Input: part model. Units: mm. Frame: model coordinates. Face numbers are marked on the shaded views. Round coordinates to 2 decimals unless told otherwise and drop trailing zeros. Write each loop counter-clockwise with the first axis right and the second up, starting at its lowest first coordinate (ties: lowest second). Pieces come first, ordered by that corner, then holes. Notation, with made-up numbers: (-30, 82) -> (9, 82) arc R17 ccw to (9, 101) -> close; hole circle Ø2 at (17, -16). An arc over 180 degrees is marked (long way). Write item = value, one per line. Start each with the question number.
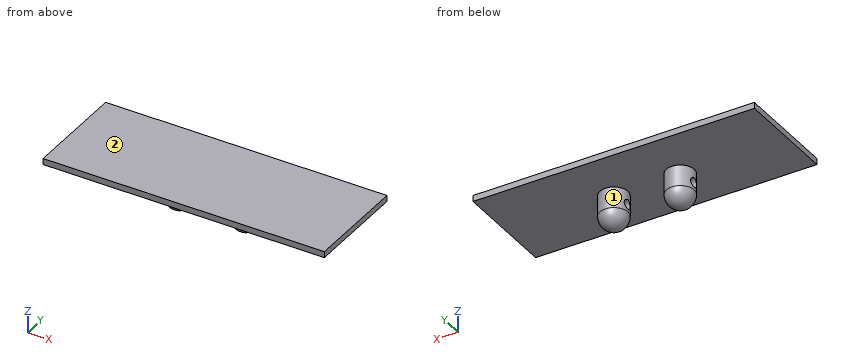
```python
from build123d import *

# Parameters (mm, degrees)
F0_W      = 88
F0_H      = 37
F1_DEPTH  = 1.75
F2_W      = 80.5
F2_H      = 29.5
F3_DEPTH  = 1.5
F4_R      = 4
F5_DEPTH  = 10
F6_R      = 4
F7_R      = 1.35
F8_DEPTH  = 88.001
F9_R      = 3
F10_DEPTH = 25


with BuildPart() as f1:
    # F0 (on Top) → F1 (new body)
    with BuildSketch(Plane.XY):
        with Locations((-44, 18.5)):
            Rectangle(F0_W, F0_H)
    extrude(amount=F1_DEPTH)

    # F2 (on face) → F3 (join)
    with BuildSketch(Plane.XY.offset(1.75)):
        with Locations((-44, 18.5)):
            Rectangle(F2_W, F2_H)
    extrude(amount=F3_DEPTH)

    # F4 (on face) → F5 (join)
    with BuildSketch(Plane(origin=(0, 0, 0), x_dir=(1, 0, 0), z_dir=(0, 0, -1))):
        with Locations((-53.5, -17.5)):
            Circle(F4_R)
        with Locations((-34.5, -17.5)):
            Circle(F4_R)
    extrude(amount=F5_DEPTH)

    # F6
    f6_edges = [f1.edges().sort_by_distance(p)[0] for p in [
        (-57.5, 17.5, -10),
        (-38.5, 17.5, -10),
    ]]
    fillet(f6_edges, radius=F6_R)

    # F7 (on face) → F8 (cut, through all)
    with BuildSketch(Plane.YZ):
        with Locations((17.5, -3.85)):
            Circle(F7_R)
    extrude(amount=-F8_DEPTH, mode=Mode.SUBTRACT)

    # F9
    f9_edges = [f1.edges().sort_by_distance(p)[0] for p in [
        (-88, 0, 0.875),
        (-88, 37, 0.875),
        (0, 37, 0.875),
        (0, 0, 0.875),
    ]]
    fillet(f9_edges, radius=F9_R)

    # F2 (on face) → F10 (intersect)
    with BuildSketch(Plane.XY.offset(1.75)):
        with Locations((-44, 18.5)):
            Rectangle(F2_W, F2_H)
    extrude(amount=-F10_DEPTH, mode=Mode.INTERSECT)


solid = f1.part
```
1. Section D-D (y = 8.5). Output: boundary loops of the cut face in (x, z).
2. Pin query (flat end, axial travel): P1, Ø5, axis at y = 27, z = -1, coming from the -X side; P2, Ø4, axis at x = -63.5, y = 11, coming from the -Z side; P3, Ø4.5, axis at y = 17.5, z = -3.85, coming from the -X side. Return the tip coordinate at first contact, or that it passes through.
3. Line query: line 1 along X through (y, z) = (19.75, -5); line 2 along X through (y, z) = (14.25, -5.75); line 3 along Y through (x, z) = (-54, -3.85). Output: solid intervals per line, ascending.
4. Section C-C (z = -3.85). Output: boundary loops of the cut face in (x, y).
5. Section B-B (z = -0.75). Output: boundary loops of the cut face in (x, y).
6. Mould query, pull axis X, two halves, no side actions, for the marked faces 1 and 2. Classes: pulls with the +X half, pulls with the -X half, needs draft (parallel to the pull), parting line crosses it, or undercut.
7. Section A-A (x = -34.5). Output: boundary loops of the cut face in (y, z), then the cut area to 3 significant figures.
Check sheet entries:
q1.outline = (-84.25, 0) -> (-3.75, 0) -> (-3.75, 1.75) -> (-84.25, 1.75) -> close
q2.P1 = -84.25
q2.P2 = 0
q2.P3 = -57.5
q3.line_1 = -56.81 to -50.19, -37.81 to -31.19
q3.line_2 = -55.83 to -51.17, -36.83 to -32.17
q3.line_3 = 13.53 to 16.15, 18.85 to 21.47
q4.outline = (-57.27, 16.15) arc R4 ccw to (-49.73, 16.15) -> close; (-57.27, 18.85) -> (-49.73, 18.85) arc R4 ccw to start; (-38.27, 16.15) arc R4 ccw to (-30.73, 16.15) -> close; (-38.27, 18.85) -> (-30.73, 18.85) arc R4 ccw to start
q5.outline = circle Ø8 at (-53.5, 17.5); circle Ø8 at (-34.5, 17.5)
q6.face_1 = undercut
q6.face_2 = needs draft
q7.outline = (3.75, 0) -> (13.5, 0) -> (13.5, -6) arc R4 ccw to (21.5, -6) -> (21.5, 0) -> (33.25, 0) -> (33.25, 1.75) -> (3.75, 1.75) -> close; hole circle Ø2.7 at (17.5, -3.85)
q7.area = 119 mm2
